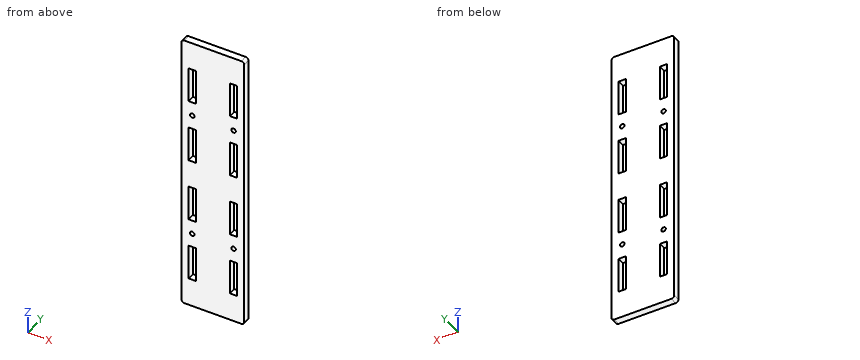
Autodesk Inventor part; units mm, degrees
ref_plane "Work Plane1" through (-22, 0, 0) normal (1, 0, 0) x (0, 0, -1)
ref_plane "Work Plane2" through (0, 0, -100) normal (0, 0, -1) x (-1, 0, 0)
ref_plane "YZ Plane" through (0, 0, 0) normal (1, 0, 0) x (0, 1, 0)
sketch "Sketch1" plane through (0, 0, 0) normal (0, 1, 0) x (-1, 0, 0)
  line L0 (0, 0) -> (0, -200)
  line L1 (0, -200) -> (44, -200)
  line L2 (44, -200) -> (44, 0)
  line L3 (44, 0) -> (0, 0)
  dimension "d0" = 200
  dimension "d1" = 44
extrude "Extrusion1" add sketch "Sketch1" along normal blind 5
sketch "Sketch2" plane through (0, 5, 0) normal (0, 1, 0) x (1, 0, 0)
  line L0 (-10, 8) -> (-10, 208)
  line L1 (-10, 208) -> (-30, 208)
  line L2 (-30, 208) -> (-30, 8)
  line L3 (-30, 8) -> (-10, 8)
  line L4 (-10, 8) -> (-30, 208) construction
  line L5 (-10, 208) -> (-30, 8) construction
  line L6 (0, 200) -> (-44, 200)
  line L7 (-44, 0) -> (0, 0)
  line L8 (0, 0) -> (0, 200)
  line L9 (-35, 0) -> (-35, 200)
  line L10 (-5, 0) -> (-5, 200)
  line L11 (-35, 10) -> (-30, 10)
  line L12 (-10, 20) -> (-5, 20)
  line L13 (-35, 35) -> (-30, 35)
  line L14 (-10, 45) -> (-5, 45)
  line L15 (-35, 55) -> (-30, 55)
  line L16 (-10, 65) -> (-5, 65)
  line L17 (-35, 80) -> (-30, 80)
  line L18 (-10, 90) -> (-5, 90)
  point P0 (-20, 108)
  dimension "d4" = 200
  dimension "d5" = 20
  dimension "d6" = 108
  dimension "d8" = 5
  dimension "d9" = 5
  dimension "d14" = 10
  dimension "d15" = 25
  dimension "d16" = 20
  dimension "d17" = 25
  dimension "d18" = 20
  dimension "d19" = 25
  dimension "d20" = 20
  dimension "d21" = 25
  dimension "d41" = 5
extrude "Extrusion2" cut sketch "Sketch2" against normal blind 5 contours L0 L14 L10 L12 | L0 L18 L10 L16
ref_plane "Work Plane1" through (-22, 0, 0) normal (1, 0, 0) x (0, 0, -1)
ref_plane "Work Plane2" through (0, 0, -100) normal (0, 0, -1) x (-1, 0, 0)
mirror "Mirror1" about plane through (-22, 0, 0) normal (1, 0, 0) of "Extrusion2"
mirror "Mirror2" about plane through (0, 0, -100) normal (0, 0, -1) of "Extrusion2", "Mirror1"
sketch "Sketch5" plane through (0, 5, 0) normal (0, 1, 0) x (1, 0, 0)
  circle A0 centre (-7.5, 55) radius 1.6
  line L0 (-10, 45) -> (-5, 45)
  line L1 (-5, 45) -> (-5, 20)
  line L2 (0, 0) -> (0, 200)
  line L3 (0, 100) -> (-44, 100)
  line L4 (-44, 200) -> (-44, 0)
  line L5 (0, 200) -> (-44, 200)
  line L6 (-22, 200) -> (-22, 0)
  line L7 (-44, 0) -> (0, 0)
  circle A1 centre (-7.5, 145) radius 1.6
  circle A2 centre (-36.5, 55) radius 1.6
  circle A3 centre (-36.5, 145) radius 1.6
  dimension "d42" = 3.2
  dimension "d43" = 10
  dimension "d44" = 2.5
extrude "Extrusion4" cut sketch "Sketch5" against normal blind 5 contours A0 | A1 | A2 | A3
fillet "Fillet1" radius 2 4 edges at (-44, 2.5, 0) (0, 2.5, 0) (0, 2.5, -200) (-44, 2.5, -200)
properties part number "BatPlate" material "ABS Plastic"
The listing builds one solid part. Answer for the finished solid, in the listing's coordinates (mm). Give positions to 0.01 mm unless a question says otherwise; leave off trailing zeros. Write each loop counter-clockwise with the first axis right and the second up, starting at its lowest first coordinate (ties: lowest second). Pieces come first, ordered by that corner, then holes. Notation, with made-up numbers: (19.25, -23) - (55.25, -23) arc R20 ccw to (55.25, -10) - close; hole circle Ø3 at (24, 0.25). An arc over 180 degrees is marked (long way). Use a Markdown table: item, result.
1. Find the intervals of material crossed by probe 1 along X at (y, z) = (1.35, -73.5); probe 2 along X at (y, z) = (2.05, -145), in increasing order. Write a range as from..to.
Values follow:
| item | result |
|---|---|
| probe 1 | x = -44..-39, -34..-10, -5..0 |
| probe 2 | x = -44..-38.1, -34.9..-9.1, -5.9..0 |
2. Section B-B on y = 4.05 is taken. Count the separate pieces of the cut face and the enclosed holes in it, plus the area to 3 significant figures.
Values follow:
| item | result |
|---|---|
| separate pieces | 1 |
| enclosed holes | 12 |
| area | 7,760 mm² |
3. Section A-A on z = -115.5 is taken. Write down the section's boundary in (x, y).
Values follow:
| item | result |
|---|---|
| outline | (-44, 0) - (-39, 0) - (-39, 5) - (-44, 5) - close; (-34, 0) - (-10, 0) - (-10, 5) - (-34, 5) - close; (-5, 0) - (0, 0) - (0, 5) - (-5, 5) - close |
